CAD build for the part. Positions are in the model's coordinates, mm. Face numbers are marked on the shaded views. Give positions to 0.01 mm unless a question says otherwise; leave off trailing zeros. Write each loop counter-clockwise with the first axis right and the second up, starting at its lowest first coordinate (ties: lowest second). Pieces come first, ordered by that corner, then holes. Notation, with made-up numbers: (-2.5, 73) - (5.5, 73) arc R13 ccw to (5.5, 84) - close; hole circle Ø1 at (-28.5, 47). An arc over 180 degrees is marked (long way). Answer as a JSON object with one key per item and string values.
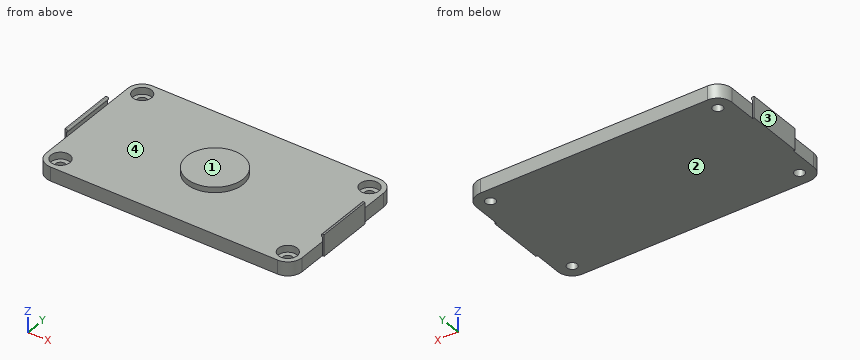
from build123d import *

# Parameters (mm, degrees)
SKETCH1_R           = 2.2098
BOSS_EXTRUDE1_DEPTH = 6.223
SKETCH2_R           = 4.2164
CUT_EXTRUDE1_DEPTH  = 3.048
SKETCH4_W           = 0.762
SKETCH4_H           = 25.4
BOSS_EXTRUDE2_DEPTH = 3.1115
BOSS_EXTRUDE3_DEPTH = 25.4
SKETCH6_R           = 12.573
BOSS_EXTRUDE4_DEPTH = 2.413


with BuildPart() as part:
    # Sketch1 → Boss-Extrude1 (new body)
    with BuildSketch(Plane.XY):
        with BuildLine():
            Line((-50.8, -31.75), (50.8, -31.75))
            ThreePointArc((50.8, -31.75), (55.290128061, -29.890128061), (57.15, -25.4))
            Line((57.15, -25.4), (57.15, 25.4))
            ThreePointArc((57.15, 25.4), (55.290128061, 29.890128061), (50.8, 31.75))
            Line((50.8, 31.75), (-50.8, 31.75))
            ThreePointArc((-50.8, 31.75), (-55.290128061, 29.890128061), (-57.15, 25.4))
            Line((-57.15, 25.4), (-57.15, -25.4))
            ThreePointArc((-57.15, -25.4), (-55.290128061, -29.890128061), (-50.8, -31.75))
        make_face()
        with Locations((-50.8, -25.4)):
            Circle(SKETCH1_R, mode=Mode.SUBTRACT)
        with Locations((-50.8, 25.4)):
            Circle(SKETCH1_R, mode=Mode.SUBTRACT)
        with Locations((50.8, 25.4)):
            Circle(SKETCH1_R, mode=Mode.SUBTRACT)
        with Locations((50.8, -25.4)):
            Circle(SKETCH1_R, mode=Mode.SUBTRACT)
    extrude(amount=BOSS_EXTRUDE1_DEPTH)

    # Sketch2 → Cut-Extrude1 (cut)
    with BuildSketch(Plane.XY.offset(6.223)):
        with Locations((-50.8, 25.4)):
            Circle(SKETCH2_R)
        with Locations((50.8, 25.4)):
            Circle(SKETCH2_R)
        with Locations((50.8, -25.4)):
            Circle(SKETCH2_R)
        with Locations((-50.8, -25.4)):
            Circle(SKETCH2_R)
    extrude(amount=-CUT_EXTRUDE1_DEPTH, mode=Mode.SUBTRACT)

    # Sketch4 → Boss-Extrude2 (add)
    with BuildSketch(Plane.XY):
        with Locations((-57.531, 0)):
            Rectangle(SKETCH4_W, SKETCH4_H)
        with Locations((57.531, 0)):
            Rectangle(SKETCH4_W, SKETCH4_H)
    extrude(amount=BOSS_EXTRUDE2_DEPTH)

    # Sketch5 → Boss-Extrude3 (add)
    with BuildSketch(Plane.XZ.offset(12.7)):
        with BuildLine():
            Line((-57.277, 3.1115), (-57.912, 3.1115))
            Line((-57.912, 3.1115), (-57.912, 9.525))
            Line((-57.912, 9.525), (-57.277, 9.525))
            ThreePointArc((-57.277, 9.525), (-56.642, 8.89), (-57.277, 8.255))
            Line((-57.277, 8.255), (-57.277, 3.1115))
        make_face()
        with BuildLine():
            Line((57.912, 9.525), (57.277, 9.525))
            ThreePointArc((57.277, 9.525), (56.642, 8.89), (57.277, 8.255))
            Line((57.277, 8.255), (57.277, 3.1115))
            Line((57.277, 3.1115), (57.912, 3.1115))
            Line((57.912, 3.1115), (57.912, 9.525))
        make_face()
    extrude(amount=-BOSS_EXTRUDE3_DEPTH)

    # Sketch6 → Boss-Extrude4 (add)
    with BuildSketch(Plane.XY.offset(6.223)):
        Circle(SKETCH6_R)
    extrude(amount=BOSS_EXTRUDE4_DEPTH)


solid = part.part
(1) Flat gauge pins, fed straight in: P1, Ø4, axis at x = -51, y = 26.5, coming from the +Z side (3 decimals); P2, Ø12.5, axis at x = -4.5, y = -5, coming from the +Z side; P3, Ø9.5, axis at x = -50.5, y = -26.5, coming from the +Z side. Where does each tip first touch, or does it go through?
Answer key:
{"P1": "stops at z = 3.175", "P2": "stops at z = 8.64", "P3": "stops at z = 6.22"}
(2) Probe L1, parallel to X at y = -25.4, z = 0.7; L2, parallel to Y at x = 50.8, z = 1.9. List the from-to ranges inside material, lowest first. Write a range as [from, to].
Answer key:
{"L1": "x = [-57.15, -53.01], [-48.59, 48.59], [53.01, 57.15]", "L2": "y = [-31.75, -27.61], [-23.19, 23.19], [27.61, 31.75]"}
(3) Pull direction X, two halves, no side cores. Call the marked faces 1, 2, 3 and 4: pulls with the +X half, pulls with the -X half, needs draft (parallel to the pull), parting line crosses it, or undercut.
Answer key:
{"face 1": "undercut", "face 2": "needs draft", "face 3": "pulls with the -X half", "face 4": "undercut"}
(4) Saw through at C-C, the plane x = 25. Give the cut face in (y, z), and give its area (3 significant figures).
Answer key:
{"outline": "(-31.75, 0) - (31.75, 0) - (31.75, 6.22) - (-31.75, 6.22) - close", "area": "395 mm²"}
(5) Saw through at A-A, the plane y = 26.5. Give the cut face in (x, z) (3 decimals), and give its area (3 significant figures).
Answer key:
{"outline": "(-57.054, 0) - (-52.717, 0) - (-52.717, 3.175) - (-54.87, 3.175) - (-54.87, 6.223) - (-57.054, 6.223) - close; (-48.883, 0) - (48.883, 0) - (48.883, 3.175) - (46.73, 3.175) - (46.73, 6.223) - (-46.73, 6.223) - (-46.73, 3.175) - (-48.883, 3.175) - close; (52.717, 0) - (57.054, 0) - (57.054, 6.223) - (54.87, 6.223) - (54.87, 3.175) - (52.717, 3.175) - close", "area": "636 mm²"}
